Autodesk Inventor part; units mm, degrees
ref_plane "YZ Plane" through (0, 0, 0) normal (1, 0, 0) x (0, 1, 0)
ref_plane "XZ Plane" through (0, 0, 0) normal (0, 1, 0) x (-1, 0, 0)
ref_plane "XY Plane" through (0, 0, 0) normal (0, 0, 1) x (1, 0, 0)
sketch "Sketch1" plane through (0, 0, 0) normal (0, 0, 1) x (1, 0, 0)
  circle A0 centre (0, 0) radius 8.5
  line L0 (20, 8.5) -> (20, -56.5)
  line L1 (20, -56.5) -> (-20, -56.5)
  line L2 (-20, -56.5) -> (-20, 8.5)
  arc A1 (20, 8.5) -> (-20, 8.5) centre (0, 0) ccw
  point P0 (0, 8.5)
  dimension "d0" = 17
  dimension "d1" = 65
  dimension "d3" = 20
  dimension "d4" = 8.5
extrude "Extrusion1" add sketch "Sketch1" along normal blind 6
fillet "Fillet1" radius 3 2 edges at (20, 8.5, 3) (-20, 8.5, 3)
properties part number "mdf_support"
The model under review builds one solid part; all positions refer to its coordinate system, in mm. Round coordinates to 2 decimals unless told otherwise and drop trailing zeros. Order: outer loops, then holes, each group sorted by start corner. A loop starts at its lowest first (then second) coordinate and runs counter-clockwise, first axis right, second up. Notation, with made-up numbers: (-32.75, 69) - (13.25, 69) arc R12 ccw to (13.25, 77) - close; hole circle Ø5 at (48.5, 13.25). An arc over 180 degrees is marked (long way). Use one line per item in the form item = value.
Q1. To check wall thickness, follow line 1 (Y direction, x = 0, z = 4.4); line 2 (Y direction, x = 7.5, z = 1.15); line 3 (X direction, y = -6, z = 4.3). State the ranges of each line that lie inside material, in increasing order.
Response values:
line_1 = -56.5 to -8.5, 8.5 to 21.73
line_2 = -56.5 to -4, 4 to 20.4
line_3 = -20 to -6.02, 6.02 to 20
Q2. Add section A-A on y = 0. Give the boundary of the cut face in (x, z), then the cut area to 3 significant figures.
Response values:
outline = (-20, 0) - (-8.5, 0) - (-8.5, 6) - (-20, 6) - close; (8.5, 0) - (20, 0) - (20, 6) - (8.5, 6) - close
area = 138 mm^2
Q3. Mouldability with a two-part tool opening along X and no side actions: class faces 1 (the flat face through (-20, -25, 3)), 2 (the cylindrical face through (4.57, -7.167, 2.958)), 3 (the flat face through (0, -56.5, 3)), 4 (the cylindrical face through (-0.35, 21.73, 2.96)) as pulls with the +X half, pulls with the -X half, needs draft (parallel to the pull), parting line crosses it, or undercut.
Response values:
face_1 = pulls with the -X half
face_2 = undercut
face_3 = needs draft
face_4 = parting line crosses it
Q4. Add section D-D on y = 17.5. Give the boundary of the cut face in (x, z).
Response values:
outline = (-12.88, 0) - (12.88, 0) - (12.88, 6) - (-12.88, 6) - close
Q5. Add section C-C on z = 1.85. Give the boundary of the cut face in (x, y).
Response values:
outline = (-20, -56.5) - (20, -56.5) - (20, 7.87) arc R3 ccw to (19.72, 9.12) arc R21.73 ccw to (-19.72, 9.12) arc R3 ccw to (-20, 7.87) - close; hole circle Ø17 at (0, 0)
Q6. Add section B-B on x = 0. Give the boundary of the cut face in (y, z), then the cut area to 3 significant figures.
Response values:
outline = (-56.5, 0) - (-8.5, 0) - (-8.5, 6) - (-56.5, 6) - close; (8.5, 0) - (21.73, 0) - (21.73, 6) - (8.5, 6) - close
area = 367 mm^2
